from build123d import *

# Parameters (mm, degrees)
SKETCH2_R           = 6.25
EXTRUDE1_DEPTH      = 5
SKETCH3_R           = 2
EXTRUDE2_DEPTH      = 22.5
EXTRUDE3_DEPTH      = 22.5
EXTRUDE3_DEPTH_BACK = 22.5
SKETCH4_R           = 2.25
SKETCH5_R           = 2.933820517
EXTRUDE4_DEPTH      = 0.5
LPATTERN1_COUNT     = 3
LPATTERN1_PITCH     = 2
SKETCH9_W           = 2
SKETCH9_H           = 2
EXTRUDE6_DEPTH      = 0.5
SKETCH7_R           = 3.25
CUT_EXTRUDE1_DEPTH  = 39.599438251


with BuildPart() as part:
    # Sketch2 → Extrude1 (new, symmetric)
    with BuildSketch(Plane.XY):
        Circle(SKETCH2_R)
    extrude(amount=EXTRUDE1_DEPTH, both=True)

    # Sketch3 → Extrude2 (add)
    with BuildSketch(Plane(origin=(0, 0, 0), x_dir=(-1, 0, 0), z_dir=(0, 1, 0))):
        with Locations(Location((0, 0, 0), (0, 0, 270))):
            Circle(SKETCH3_R)
    extrude(amount=EXTRUDE2_DEPTH)

    # Sketch4 → Extrude3 (add, two sides: drawn at the far end of the back side and taken through both)
    with BuildSketch(Plane(origin=(0, 0, 0), x_dir=(0, 0, -1), z_dir=(1, 0, 0)).offset(-EXTRUDE3_DEPTH_BACK)):
        with Locations((0, 22.5)):
            Circle(SKETCH4_R)
    extrude(amount=EXTRUDE3_DEPTH + EXTRUDE3_DEPTH_BACK)

    # Sketch5 → Extrude4 (add)
    with BuildSketch(Plane(origin=(12, 0, 0), x_dir=(0, 0, -1), z_dir=(1, 0, 0))):
        with Locations((0, 22.5)):
            Circle(SKETCH5_R)
    extrude4 = extrude(amount=EXTRUDE4_DEPTH)

    # LPattern1: Extrude4 ×3
    with Locations(*[(i * LPATTERN1_PITCH, 0, 0) for i in range(1, LPATTERN1_COUNT)]):
        add(extrude4)

    # Sketch9 → Extrude6 (add)
    with BuildSketch(Plane(origin=(22.5, 0, 0), x_dir=(0, 0, -1), z_dir=(1, 0, 0))):
        with Locations((0, 22.5)):
            Rectangle(SKETCH9_W, SKETCH9_H)
    extrude(amount=EXTRUDE6_DEPTH)

    # Extrude5 cone 1 section (on through the dimple's axis) → Extrude5 (revolve)
    with BuildSketch(Plane(origin=(22.5, 22.5, 0), x_dir=(0, 0, 1), z_dir=(0, 1, 0))):
        Polygon((0, 0), (0.925, 0), (0, 4.758712465), align=None)
    revolve(axis=Axis((22.5, 22.5, 0), (1, 0, 0)))

    # Sketch7 → Cut-Extrude1 (cut, through all)
    with BuildSketch(Plane.XY.offset(5)):
        Circle(SKETCH7_R)
    extrude(amount=-CUT_EXTRUDE1_DEPTH, mode=Mode.SUBTRACT)


solid = part.part
Geometry: final body of the model. Coordinates: model frame, mm. A direction names the side the tool comes from. Coordinates: 2 decimals unless noted, no trailing zeros. Order: outer loops, then holes, each group sorted by start corner. A loop starts at its lowest first (then second) coordinate and runs counter-clockwise, first axis right, second up.
(1) Draft query along Y for faces 1 (the face through (2.884, -5.545, 0.07)), 2 (the face through (3, -3, -5)), 3 (the face through (-5.49, 24.73, 0.29)), 4 (the face through (16.25, 24.97, -1.58)). Return one class per face: pulls with the +Y half, pulls with the -Y half, needs draft (parallel to the pull), parting line crosses it, or undercut.
(2) Section query D-D (y = 15). Return the cut outline in (x, z).
(3) First-contact query: pin 1 (0.6 mm diameter, centred on x = 22.5, y = 23, fed in from +Z); pin 2 (3 mm diameter, centred on x = -11, z = -2.5, fed in from -Y); pin 3 (1.5 mm diameter, centred on x = 5.5, y = 21, fed in from +Z). Flat tips, straight axial feed; report the tip coordinate or a pass-through.
(4) Access query for faces 5 (the face through (19.458, 20.304, 0.488)), 6 (the face through (12.5, 20, 1)), 7 (the face through (3, -3, 5)). Directions: +Z, -Z, +X, -X, +Y, -Y. A direction counts if a zero-diameter tool reaches every point of the face in a straight line with its end or side. Return the directions, or none.
(5) Section query C-C (z = -3.75). Return the cut outline in (x, y).
(6) Material intervals for probe 1 along Y at (x, z) = (0, -2.5); probe 2 along X at (y, z) = (1.5, -4.25); probe 3 along Y at (x, z) = (-1, 0), sorted ascending.
(7) Section query B-B (y = 0). Return the cut outline in (x, z), plus the area to 3 significant figures.
(8) Section query A-A (x = 0). Return the cut outline in (y, z).
Solution:
1. face 1: undercut
1. face 2: needs draft
1. face 3: undercut
1. face 4: parting line crosses it
2. outline: circle Ø4 at (0, 0)
3. pin 1: stops at z = 2.24
3. pin 2: stops at y = 20.48
3. pin 3: stops at z = 2.12
4. face 5: +X
4. face 6: none
4. face 7: +Z, +X, -X, +Y, -Y
5. outline: circle Ø12.5 at (0, 0); hole circle Ø6.5 at (0, 0)
6. probe 1: y = -6.25 to -3.25, 3.25 to 6.25
6. probe 2: x = -6.07 to -2.88, 2.88 to 6.07
6. probe 3: y = -6.17 to -3.09, 3.09 to 24.75
7. outline: (-6.25, -5) - (-3.25, -5) - (-3.25, 5) - (-6.25, 5) - close; (3.25, -5) - (6.25, -5) - (6.25, 5) - (3.25, 5) - close
7. area: 60.0 mm2
8. outline: (-6.25, -5) - (-3.25, -5) - (-3.25, 5) - (-6.25, 5) - close; (3.25, -5) - (6.25, -5) - (6.25, -2) - (21.47, -2) arc R2.25 ccw (long way) to (21.47, 2) - (6.25, 2) - (6.25, 5) - (3.25, 5) - close
